Input: part model. Units: mm. Frame: model coordinates. A direction names the side the tool comes from. Round coordinates to 2 decimals unless told otherwise and drop trailing zeros. Order: outer loops, then holes, each group sorted by start corner. A loop starts at its lowest first (then second) coordinate and runs counter-clockwise, first axis right, second up. Notation, with made-up numbers: M -17,-3 L 14,-3 A20 cw 14,14 Z; hole C -34.5,59.5 d4. An arc over 180 degrees is marked long. One line per question, with ' | ' between items.
```python
from build123d import *

# Parameters (mm, degrees)
BOSS_EXTRUDE1_DEPTH = 680
HOLE1_D             = 6.5


with BuildPart() as part:
    # Sketch1 → Boss-Extrude1 (new body)
    with BuildSketch(Plane.XY):
        with BuildLine():
            Line((-40, -24), (-40, 24))
            ThreePointArc((-40, 24), (-38.242640687, 28.242640687), (-34, 30))
            Line((-34, 30), (34, 30))
            ThreePointArc((34, 30), (38.242640687, 28.242640687), (40, 24))
            Line((40, 24), (40, -24))
            ThreePointArc((40, -24), (38.242640687, -28.242640687), (34, -30))
            Line((34, -30), (-34, -30))
            ThreePointArc((-34, -30), (-38.242640687, -28.242640687), (-40, -24))
        make_face()
        with BuildLine():
            Line((-34, 27), (34, 27))
            ThreePointArc((34, 27), (36.121320344, 26.121320344), (37, 24))
            Line((37, 24), (37, -24))
            ThreePointArc((37, -24), (36.121320344, -26.121320344), (34, -27))
            Line((34, -27), (-34, -27))
            ThreePointArc((-34, -27), (-36.121320344, -26.121320344), (-37, -24))
            Line((-37, -24), (-37, 24))
            ThreePointArc((-37, 24), (-36.121320344, 26.121320344), (-34, 27))
        make_face(mode=Mode.SUBTRACT)
    extrude(amount=BOSS_EXTRUDE1_DEPTH)

    # Hole1 (through all)
    with Locations(Plane(origin=(-29, 30, 669), x_dir=(1, 0, 0), z_dir=(0, 1, 0))):
        with Locations((0, 0), (0, 38), (58, 38), (58, 0), (0, 658), (0, 620), (58, 658), (58, 620)):
            Hole(HOLE1_D / 2)


solid = part.part
```
Item 1: Section query B-B, the plane y = 14.5. Return loops of the section in (x, z), plus the area to 3 significant figures.
Report:
outline: M -40,0 L -37,0 L -37,680 L -40,680 Z; M 37,0 L 40,0 L 40,680 L 37,680 Z | area: 4,080 mm²
Item 2: Mould query, pull axis X, two halves, no side actions, for faces 3 (the flat face through (0, -27, 335)), 4 (the flat face through (0, -30, 335)), 5 (the flat face through (-40, 0, 335)). Classes: +X half, -X half, draft (parallel to the pull), parting line (faces both ways), or undercut.
Report:
face 3: undercut | face 4: draft | face 5: -X half
Item 3: Access query for faces 1 (the flat face through (37, 0, 335)), 2 (the flat face through (0, 29, 680)). Directions: +Z, -Z, +X, -X, +Y, -Y. A direction counts if a zero-diameter tool reaches every point of the face in a straight line with its end or side. Return the directions, or none.
Report:
face 1: +Z, -Z | face 2: +Z, +X, -X, +Y, -Y
Item 4: Section query A-A, the plane x = -5. Return loops of the section in (y, z).
Report:
outline: M -30,0 L -27,0 L -27,680 L -30,680 Z; M 27,0 L 30,0 L 30,680 L 27,680 Z
Item 5: Section query C-C, the plane z = 312. Return loops of the section in (x, y).
Report:
outline: M -40,-24 A6 ccw -34,-30 L 34,-30 A6 ccw 40,-24 L 40,24 A6 ccw 34,30 L -34,30 A6 ccw -40,24 Z; hole M -37,-24 A3 ccw -34,-27 L 34,-27 A3 ccw 37,-24 L 37,24 A3 ccw 34,27 L -34,27 A3 ccw -37,24 Z
Item 6: First-contact query: pin 1 (8.5 mm diameter, centred on x = 29, z = 669, fed in from +Y); pin 2 (5 mm diameter, centred on x = 29, z = 49, fed in from +Y). Flat tips, straight axial feed; report the tip coordinate or a pass-through.
Report:
pin 1: y = 30 | pin 2: through
Item 7: Line query: line 1 along Z through (x, y) = (29, -28.1); line 2 along X through (y, z) = (-13, 69); line 3 along Y through (x, z) = (-7, 518.5). Output: solid intervals per line, ascending. Write a range as from..to.
Report:
line 1: 0..7.75, 14.25..45.75, 52.25..627.75, 634.25..665.75, 672.25..680 | line 2: -40..-37, 37..40 | line 3: -30..-27, 27..30
